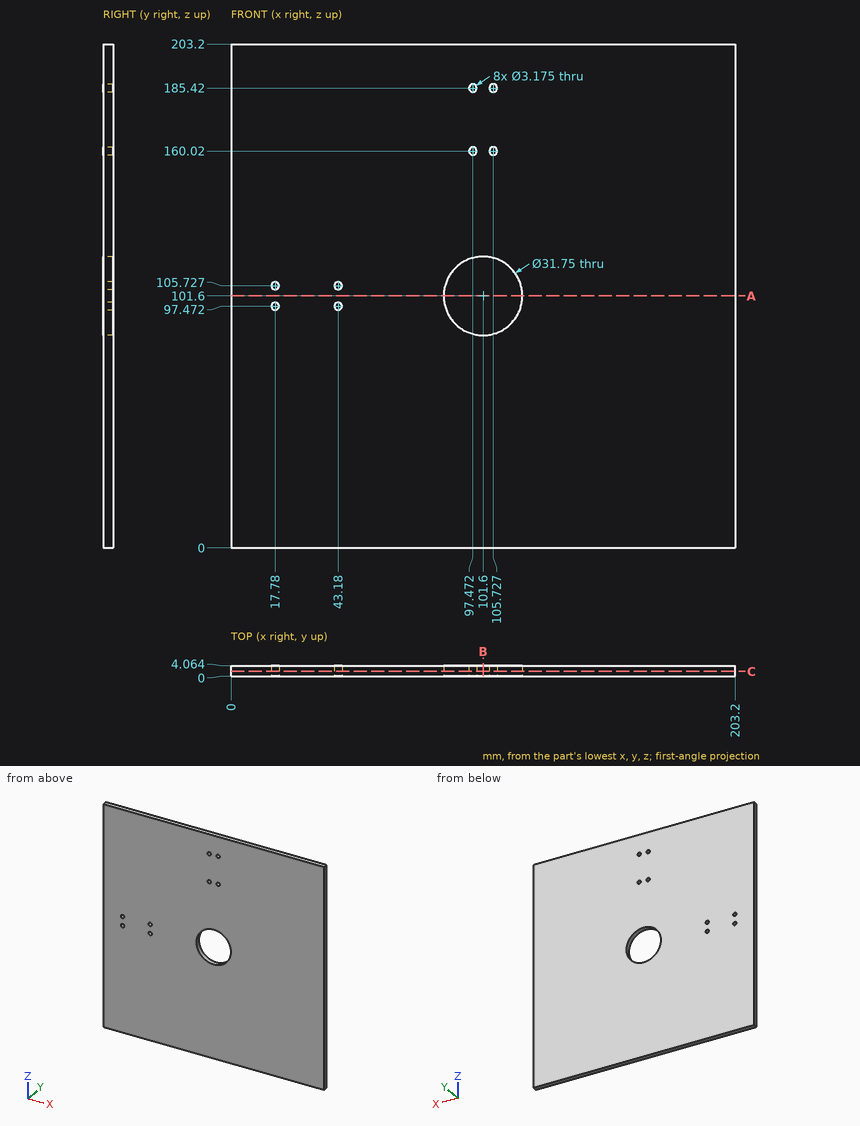
The drawing under review shows one solid part. Ordinate dimensions are in mm from its lowest x, y, z. Give positions to 0.01 mm unless a question says otherwise; leave off trailing zeros. Order: outer loops, then holes, each group sorted by start corner. A loop starts at its lowest first (then second) coordinate and runs counter-clockwise, first axis right, second up. Notation, with made-up numbers: M 36,-28.5 L 64,-28.5 A18 cw 64,-18.5 Z; hole C 75.25,-26.5 d5. An arc over 180 degrees is marked long. Answer in a Markdown table with one row per item. Add a question column.
1. Add section B-B on x = 101.6. State the section outline as (y, z) points (1 decimal).
2. Add section A-A on z = 101.6. State the section outline as (x, y) points (1 decimal).
3. Add section C-C on y = 1.9. Count the separate pieces of the cut face and the enclosed holes in it, plus the area to 3 significant figures.
4. To check wall thickness, follow line 1 along X through (y, z) = (2.2, 185.42) (1 decimal); line 2 along X through (y, z) = (3.55, 105.5). State the ranges of each line that lie inside material, in increasing order.
The answers:
| question | item | result |
|---|---|---|
| 1 | outline | M 0,0 L 4.1,0 L 4.1,85.7 L 0,85.7 Z; M 0,117.5 L 4.1,117.5 L 4.1,203.2 L 0,203.2 Z |
| 2 | outline | M 0,0 L 85.7,0 L 85.7,4.1 L 0,4.1 Z; M 117.5,0 L 203.2,0 L 203.2,4.1 L 117.5,4.1 Z |
| 3 | separate pieces | 1 |
| 3 | enclosed holes | 9 |
| 3 | area | 40,400 mm2 |
| 4 | line 1 | 0 to 95.9, 99.1 to 104.1, 107.3 to 203.2 |
| 4 | line 2 | 0 to 16.21, 19.35 to 41.61, 44.75 to 86.21, 116.99 to 203.2 |
